```python
from build123d import *

# Parameters (mm, degrees)
F1_DEPTH = 2.5
F2_R     = 2.6
F2_R_2   = 1.25
F3_DEPTH = 3.8
F4_DEPTH = 25
F5_R     = 0.5


with BuildPart() as f1:
    # F0 (on Top) → F1 (new body)
    with BuildSketch(Plane.XY):
        Polygon((-1.558846, -2.7), (1.558846, -2.7), (3.117691, 0), (1.558846, 2.7), (-1.558846, 2.7), (-3.117691, 0), align=None)
    extrude(amount=F1_DEPTH)

    # F2 (on face) → F3 (join)
    with BuildSketch(Plane(origin=(0, 0, 0), x_dir=(1, 0, 0), z_dir=(0, 0, -1))):
        Circle(F2_R)
        Circle(F2_R_2, mode=Mode.SUBTRACT)
    extrude(amount=-F3_DEPTH)

    # F2 (on face) → F4 (cut)
    with BuildSketch(Plane(origin=(0, 0, 0), x_dir=(1, 0, 0), z_dir=(0, 0, -1))):
        Circle(F2_R_2)
    extrude(amount=-F4_DEPTH, mode=Mode.SUBTRACT)

    # F5
    f5_edges = [f1.edges().sort_by_distance(p)[0] for p in [
        (-2.6, 0, 3.8),
    ]]
    fillet(f5_edges, radius=F5_R)


solid = f1.part
```
The model under review builds one solid part; all positions refer to its coordinate system, in mm. A direction names the side the tool comes from. Give positions to 0.01 mm unless a question says otherwise; leave off trailing zeros. Write each loop counter-clockwise with the first axis right and the second up, starting at its lowest first coordinate (ties: lowest second). Pieces come first, ordered by that corner, then holes. Notation, with made-up numbers: M 70.25,-2 L 127.25,-2 A9 cw 127.25,2 Z; hole C 80.5,38 d7. An arc over 180 degrees is marked long. Write item = value, one per line. Start each with the question number.
Q1. For line 1 (Y direction, x = 0, z = 0.75); line 2 (Y direction, x = 0, z = 2.55); line 3 (X direction, y = -0.85, z = 2.55), list the stretches that pass through material, from the lowest coordinate up.
Q2. Clearance check with a flat-ended pin moving along its axis: pin 1 (1.5 mm diameter, centred on y = -0.5, z = 2, fed in from +X). State where the tip first meets the part, or that it passes through.
Q3. We need section B-B (x = 0). State the section outline as (y, z) points, plus the area to 3 significant figures.
Q4. We need section A-A (z = 1.5). State the section outline as (x, y) points.
Q5. Mouldability with a two-part tool opening along X and no side actions: class faces 1 (the face through (-2.327, 1.369, 1.232)), 2 (the face through (0, -2.7, 1)), 3 (the face through (-0.27, 1.22, 1.87)) as released by +X, released by -X, zero draft, split by the parting line, or undercut.
Q6. Machinability: for faces 4 (the face through (1, 1, 0)), 5 (the face through (-0.338, -2.578, 2.894)), which of the approach directions +Z, -Z, +X, -X, +Y, -Y give a long, thin tool a straight path to every point of the face, cutting with its end or side? Answer none if there is none.
Result set:
q1.line_1 = -2.7 to -1.25, 1.25 to 2.7
q1.line_2 = -2.6 to -1.25, 1.25 to 2.6
q1.line_3 = -2.46 to -0.92, 0.92 to 2.46
q2.pin_1 = 3.12
q3.outline = M -2.7,0 L -1.25,0 L -1.25,3.8 L -2.1,3.8 A0.5 ccw -2.6,3.3 L -2.6,2.5 L -2.7,2.5 Z; M 1.25,0 L 2.7,0 L 2.7,2.5 L 2.6,2.5 L 2.6,3.3 A0.5 ccw 2.1,3.8 L 1.25,3.8 Z
q3.area = 10.7 mm2
q4.outline = M -3.12,0 L -1.56,-2.7 L 1.56,-2.7 L 3.12,0 L 1.56,2.7 L -1.56,2.7 Z; hole C 0,0 d2.5
q5.face_1 = released by -X
q5.face_2 = zero draft
q5.face_3 = undercut
q6.face_4 = -Z, +X, -X, +Y, -Y
q6.face_5 = +Z
